Check sheet for the modelled part. Datum: model origin and axes. Units: mm. A direction names the side the tool comes from. Round coordinates to 2 decimals unless told otherwise and drop trailing zeros. Loops run counter-clockwise (first coordinate to the right, second up) from the corner with the lowest first, then second, coordinate; pieces in that order, holes last. Notation, with made-up numbers: (29, 32) -> (54, 32) arc R26 ccw to (54, 51) -> close; hole circle Ø9 at (89, -6). An arc over 180 degrees is marked (long way). Return JSON: item names as keys, results as strings.
from build123d import *

# Parameters (mm, degrees)
F0_R     = 6
F0_R_2   = 4.8
F1_DEPTH = 80
F3_DEPTH = 12.5
F5_DEPTH = 15
F6_R     = 4.8
F7_DEPTH = 2
F8_R     = 0.5
F9_SIZE  = 0.5


with BuildPart() as f1:
    # F0 (on Top) → F1 (new body)
    with BuildSketch(Plane.XY):
        Circle(F0_R)
        Circle(F0_R_2, mode=Mode.SUBTRACT)
    extrude(amount=F1_DEPTH)

    # F2 (on Right) → F3 (cut, symmetric)
    with BuildSketch(Plane.YZ):
        Polygon((-6.6873627901, 30), (-6.6873627901, 20), (-3.1873627901, 20), align=None)
    extrude(amount=F3_DEPTH, both=True, mode=Mode.SUBTRACT)

    # F4 (on face) → F5 (join)
    with BuildSketch(Plane.XY.offset(20)):
        with BuildLine():
            Line((-3.5889717809, -3.1873627901), (3.5889717809, -3.1873627901))
            ThreePointArc((3.5889717809, -3.1873627901), (0, 4.8), (-3.5889717809, -3.1873627901))
        make_face()
    extrude(amount=-F5_DEPTH)

    # F6 (on face) → F7 (join)
    with BuildSketch(Plane.XY.offset(80)):
        Circle(F6_R)
    extrude(amount=-F7_DEPTH)

    # F8
    f8_edges = [f1.edges().sort_by_distance(p)[0] for p in [
        (-6, 0, 0),
    ]]
    fillet(f8_edges, radius=F8_R)

    # F9
    f9_edges = [f1.edges().sort_by_distance(p)[0] for p in [
        (-6, 0, 80),
    ]]
    chamfer(f9_edges, length=F9_SIZE)


solid = f1.part
Q1. Section check B-B (z = 8.5). Record the boundary of the cut face in (x, y).
Results list:
{"outline": "circle Ø12 at (0, 0); hole (-3.59, -3.19) arc R4.8 ccw to (3.59, -3.19) -> close"}
Q2. Section check C-C (x = 0). Record the boundary of the cut face in (y, z), then the cut area to 3 significant figures.
Results list:
{"outline": "(-6, 0.5) arc R0.5 ccw to (-5.5, 0) -> (-4.8, 0) -> (-4.8, 20) -> (-6, 20) -> close; (-6, 28.04) -> (-4.8, 24.61) -> (-4.8, 78) -> (4.8, 78) -> (4.8, 20) -> (-3.19, 20) -> (-3.19, 5) -> (4.8, 5) -> (4.8, 0) -> (5.5, 0) arc R0.5 ccw to (6, 0.5) -> (6, 79.5) -> (5.5, 80) -> (-5.5, 80) -> (-6, 79.5) -> close", "area": "323 mm^2"}
Q3. Draft check along Y on faces 4 (the cylindrical face through (-0.78, 5.95, 39.45)), 5 (the flat face through (0, 0, 80)), 6 (the cylindrical face through (-0.62, 4.76, 48.59)). Enter one of: released by +Y, released by -Y, zero draft, split by the parting line, or undercut.
Results list:
{"face 4": "split by the parting line", "face 5": "zero draft", "face 6": "undercut"}
Q4. Go/stop test with flat-tipped pins: pin 1 (5 mm diameter, centred on x = 0.5, z = 36.5, fed in from +Y); pin 2 (2 mm diameter, centred on x = -1.5, y = 1.5, fed in from -Z); pin 3 (3 mm diameter, centred on x = 2, z = 9.5, fed in from -Y). Record where each tip stops, or that it passes through.
Results list:
{"pin 1": "y = 6", "pin 2": "z = 5", "pin 3": "y = -5.98"}
Q5. Section check A-A (y = 0). Record the boundary of the cut face in (x, z), then the cut area to 3 significant figures.
Results list:
{"outline": "(-6, 0.5) arc R0.5 ccw to (-5.5, 0) -> (-4.8, 0) -> (-4.8, 5) -> (4.8, 5) -> (4.8, 0) -> (5.5, 0) arc R0.5 ccw to (6, 0.5) -> (6, 79.5) -> (5.5, 80) -> (-5.5, 80) -> (-6, 79.5) -> close; hole (-4.8, 20) -> (4.8, 20) -> (4.8, 78) -> (-4.8, 78) -> close", "area": "355 mm^2"}
Q6. Section check D-D (z = 48). Record the boundary of the cut face in (x, y).
Results list:
{"outline": "circle Ø12 at (0, 0); hole circle Ø9.6 at (0, 0)"}
Q7. Material ranges on line 1 (Z direction, x = -0.5, y = -2.75); line 2 (Y direction, x = 0, z = 9.25); line 3 (Y direction, x = 0, z = 64), recorded low to high.
Results list:
{"line 1": "5 to 20, 78 to 80", "line 2": "-6 to -4.8, -3.19 to 6", "line 3": "-6 to -4.8, 4.8 to 6"}
Q8. Tool access check on faces 1 (the flat face through (0, 1, 5)), 2 (the flat face through (0, 0, 78)), 3 (the flat face through (0, 5, 0)). Record the directions out of +Z, -Z, +X, -X, +Y, -Y that give a thin tool (end or side, any length) a straight path to the whole face; none if there is none.
Results list:
{"face 1": "-Z", "face 2": "none", "face 3": "-Z, +X, -X, +Y, -Y"}
